Geometry: see drawing. Coordinates: mm, zero at the bounding-box minimum. A direction names the side the tool comes from. Coordinates: 2 decimals unless noted, no trailing zeros. Order: outer loops, then holes, each group sorted by start corner. A loop starts at its lowest first (then second) coordinate and runs counter-clockwise, first axis right, second up. Notation, with made-up numbers: (23.5, -25) -> (68.5, -25) arc R21 ccw to (68.5, -3) -> close; hole circle Ø6 at (57.25, -0.5). An arc over 180 degrees is marked (long way). Use one line per item in the form item = value.
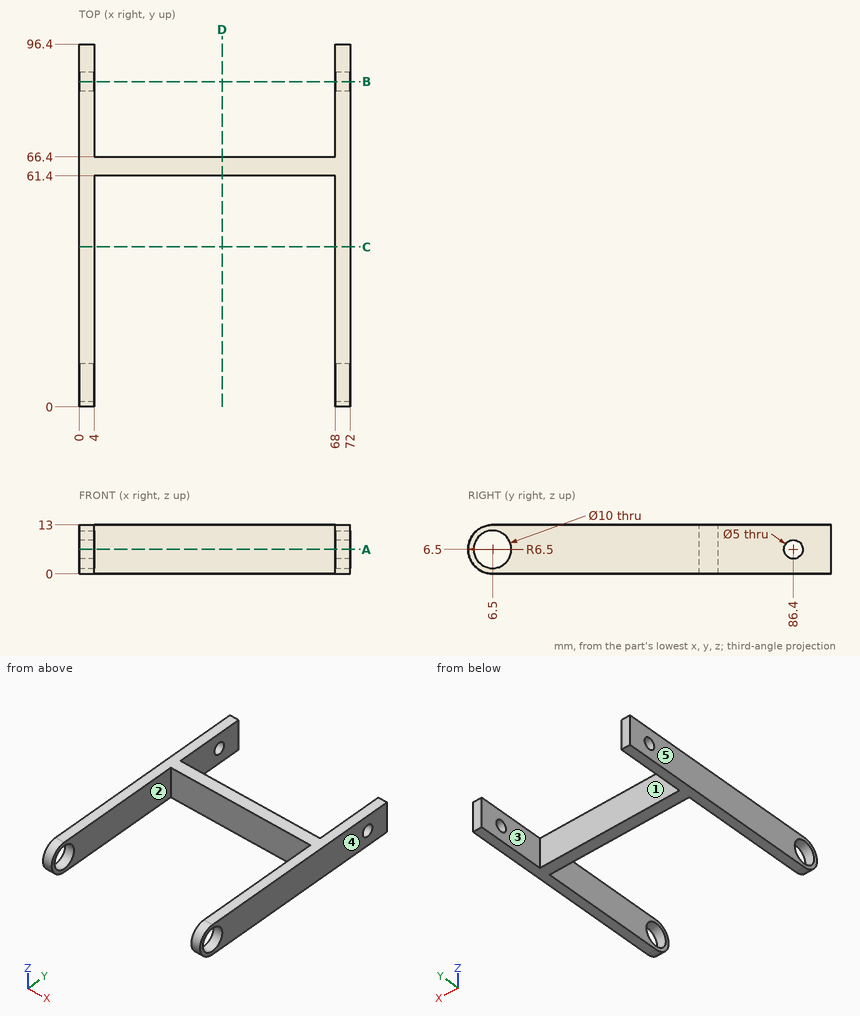
1) Pull-direction query (X, two-part tool) for the marked faces 3, 4 and 5; classes: released by +X, released by -X, zero draft, split by the parting line, or undercut.
Results found:
face_3 = undercut
face_4 = released by +X
face_5 = released by -X
2) Section D-D, the plane x = 38. Output: boundary loops of the cut face in (y, z).
Results found:
outline = (61.4, 0) -> (66.4, 0) -> (66.4, 13) -> (61.4, 13) -> close
3) Section B-B, the plane y = 86.4. Output: boundary loops of the cut face in (x, z).
Results found:
outline = (0, 0) -> (4, 0) -> (4, 4) -> (0, 4) -> close; (0, 9) -> (4, 9) -> (4, 13) -> (0, 13) -> close; (68, 0) -> (72, 0) -> (72, 4) -> (68, 4) -> close; (68, 9) -> (72, 9) -> (72, 13) -> (68, 13) -> close
4) Section A-A, the plane z = 6.5. Output: boundary loops of the cut face in (x, y).
Results found:
outline = (0, 0) -> (4, 0) -> (4, 1.5) -> (0, 1.5) -> close; (0, 11.5) -> (4, 11.5) -> (4, 61.4) -> (68, 61.4) -> (68, 11.5) -> (72, 11.5) -> (72, 83.9) -> (68, 83.9) -> (68, 66.4) -> (4, 66.4) -> (4, 83.9) -> (0, 83.9) -> close; (0, 88.9) -> (4, 88.9) -> (4, 96.4) -> (0, 96.4) -> close; (68, 0) -> (72, 0) -> (72, 1.5) -> (68, 1.5) -> close; (68, 88.9) -> (72, 88.9) -> (72, 96.4) -> (68, 96.4) -> close
5) Section C-C, the plane y = 42.5. Output: boundary loops of the cut face in (x, z).
Results found:
outline = (0, 0) -> (4, 0) -> (4, 13) -> (0, 13) -> close; (68, 0) -> (72, 0) -> (72, 13) -> (68, 13) -> close
6) Contact query for flat-ended pins moving along their axis: P1, Ø4.5, axis at y = 86.4, z = 6.5, coming from the +X side; P2, Ø4, axis at x = 21.5, z = 9, coming from the +Y side; P3, Ø2, axis at x = 11, z = 2, coming from the -Y side. Output: stop coordinate, or through.
Results found:
P1 = through
P2 = 66.4
P3 = 61.4
7) Material intervals for probe 1 along X at (y, z) = (92, 5.5); probe 2 along Z at (x, y) = (1.4, 6.5); probe 3 along Y at (x, z) = (41, 9.5), sorted ascending. Write a range as from..to.
Results found:
probe_1 = 0..4, 68..72
probe_2 = 0..1.5, 11.5..13
probe_3 = 61.4..66.4
8) Access query for the marked faces 1 and 2. Directions: +Z, -Z, +X, -X, +Y, -Y. A direction counts if a zero-diameter tool reaches every point of the face in a straight line with its end or side. Return the directions, or none.
Results found:
face_1 = +Z, -Z, +Y
face_2 = +Z, -Z, -Y
